from build123d import *

# Parameters (mm, degrees)
BOSS_EXTRUDE1_DEPTH      = 1
M2_CLEARANCE_HOLE1_D     = 2.6
M2_CLEARANCE_HOLE1_DEPTH = 1
CUT_EXTRUDE1_REACH       = 7
SKETCH15_R               = 0.75


with BuildPart() as part:
    # Sketch2 → Boss-Extrude1 (new body)
    with BuildSketch(Plane.XY):
        with BuildLine():
            Line((-5, 2.5), (5, 2.5))
            ThreePointArc((5, 2.5), (6.414213562, 1.914213562), (7, 0.5))
            Line((7, 0.5), (7, -0.5))
            ThreePointArc((7, -0.5), (6.414213562, -1.914213562), (5, -2.5))
            Line((5, -2.5), (-5, -2.5))
            ThreePointArc((-5, -2.5), (-6.414213562, -1.914213562), (-7, -0.5))
            Line((-7, -0.5), (-7, 0.5))
            ThreePointArc((-7, 0.5), (-6.414213562, 1.914213562), (-5, 2.5))
        make_face()
    extrude(amount=BOSS_EXTRUDE1_DEPTH)

    # M2 Clearance Hole1
    with Locations(Plane(origin=(0, 0, 0), x_dir=(-1, 0, 0), z_dir=(0, 0, -1))):
        with Locations((-5, 0), (5, 0)):
            Hole(M2_CLEARANCE_HOLE1_D / 2, depth=M2_CLEARANCE_HOLE1_DEPTH)

    # Sketch15 → Cut-Extrude1 (cut, up to next)
    with BuildSketch(Plane.XZ.offset(2.5), mode=Mode.PRIVATE) as cut_extrude1_sk1:
        with Locations((0, -0.5)):
            Circle(SKETCH15_R)
    cut_extrude1_tool1 = extrude(cut_extrude1_sk1.sketch, amount=-CUT_EXTRUDE1_REACH, mode=Mode.PRIVATE) & part.part
    add(cut_extrude1_tool1.solids().sort_by_distance((0, -2.5, -0.5))[0], mode=Mode.SUBTRACT)


solid = part.part
The listing builds one solid part. Answer for the finished solid, in the listing's coordinates (mm). Coordinates: 2 decimals unless noted, no trailing zeros. Write each loop counter-clockwise with the first axis right and the second up, starting at its lowest first coordinate (ties: lowest second). Pieces come first, ordered by that corner, then holes. Notation, with made-up numbers: (66.25, -3.75) - (77.25, -3.75) arc R25 ccw to (77.25, 13.25) - close; hole circle Ø11 at (88.25, -32). An arc over 180 degrees is marked (long way). Answer as CSV lines item,"result".
1. Find section C-C (x = -5.5). Give the vertices of the cut face in (y, z), plus the area to 3 significant figures.
Computed values:
outline,"(-2.44, 0) - (-1.2, 0) - (-1.2, 1) - (-2.44, 1) - close; (1.2, 0) - (2.44, 0) - (2.44, 1) - (1.2, 1) - close"
area,"2.47 mm²"
2. Find section B-B (y = 0). Give the vertices of the cut face in (x, z), plus the area to 3 significant figures.
Computed values:
outline,"(-7, 0) - (-6.3, 0) - (-6.3, 1) - (-7, 1) - close; (-3.7, 0) - (-0.56, 0) arc R0.75 cw to (0.56, 0) - (3.7, 0) - (3.7, 1) - (-3.7, 1) - close; (6.3, 0) - (7, 0) - (7, 1) - (6.3, 1) - close"
area,"8.61 mm²"
3. Find section D-D (y = -0.85). Give the vertices of the cut face in (x, z).
Computed values:
outline,"(-6.97, 0) - (-5.98, 0) - (-5.98, 1) - (-6.97, 1) - close; (-4.02, 0) - (-0.56, 0) arc R0.75 cw to (0.56, 0) - (4.02, 0) - (4.02, 1) - (-4.02, 1) - close; (5.98, 0) - (6.97, 0) - (6.97, 1) - (5.98, 1) - close"
4. Straight lines are drawn through the part: line 1 (X direction, y = 0.05, z = 0.85); line 2 (X direction, y = 0.85, z = 0.8); line 3 (Y direction, x = -5, z = 0.5). For each, find the intervals that lie inside material, in ascending order. Write a range as [from, to].
Computed values:
line 1,"x = [-7, -6.3], [-3.7, 3.7], [6.3, 7]"
line 2,"x = [-6.97, -5.98], [-4.02, 4.02], [5.98, 6.97]"
line 3,"y = [-2.5, -1.3], [1.3, 2.5]"
5. Determine the mould class of faces 1 (the cylindrical face through (-6.4, -1.93, 0.49)), 2 (the flat face through (3, 0, 0)), 3 (the cylindrical face through (0.01, -0.04, 0.25)) for opening direction X: +X half, -X half, draft (parallel to the pull), parting line (faces both ways), or undercut.
Computed values:
face 1,"-X half"
face 2,"draft"
face 3,"undercut"
6. Find section A-A (z = 0.6). Give the vertices of the cut face in (x, y).
Computed values:
outline,"(-7, -0.5) arc R2 ccw to (-5, -2.5) - (5, -2.5) arc R2 ccw to (7, -0.5) - (7, 0.5) arc R2 ccw to (5, 2.5) - (-5, 2.5) arc R2 ccw to (-7, 0.5) - close; hole circle Ø2.6 at (-5, 0); hole circle Ø2.6 at (5, 0)"
